from build123d import *

# Parameters (mm, degrees)
SKETCH2_W           = 91.08348254
SKETCH2_H           = 10.16
SKETCH2_R           = 1.75
BOSS_EXTRUDE1_DEPTH = 22.5
CUT_EXTRUDE1_DEPTH  = 88.707853004
FILLET1_R           = 5.08


with BuildPart() as part:
    # Sketch2 → Boss-Extrude1 (new, symmetric)
    with BuildSketch(Plane.XY):
        with Locations((38.619959512, 0)):
            Rectangle(SKETCH2_W, SKETCH2_H)
        with Locations(Location((38.410945338, 0, 0), (0, 0, 180))):
            Circle(SKETCH2_R, mode=Mode.SUBTRACT)
        with Locations(Location((0, 0, 0), (0, 0, 180))):
            Circle(SKETCH2_R, mode=Mode.SUBTRACT)
        with Locations(Location((78.79999988, 0, 0), (0, 0, 180))):
            Circle(SKETCH2_R, mode=Mode.SUBTRACT)
    extrude(amount=BOSS_EXTRUDE1_DEPTH, both=True)

    # Sketch3 → Cut-Extrude1 (cut, through all)
    with BuildSketch(Plane(origin=(0, 5.08, 0), x_dir=(1, 0, 0), z_dir=(0, 1, 0))):
        with BuildLine():
            Line((91.724321271, 17), (72.05824076, 17))
            ThreePointArc((72.05824076, 17), (55.05824076, 0), (72.05824076, -17))
            Line((72.05824076, -17), (91.724321271, -17))
            Line((91.724321271, -17), (91.724321271, 17))
        make_face()
        Polygon((-6.921781758, 15.097756516), (29.791957943, 18.888274186), (45.800007469, 18.888274186), (63.048045595, 22.5), (63.048045595, 41.563803389), (-6.921781758, 41.563803389), align=None)
        with BuildLine():
            Line((-35.26716372, 9.799999958), (7.296822355, 9.799999958))
            ThreePointArc((7.296822355, 9.799999958), (17.096822313, 0), (7.296822355, -9.799999958))
            Line((7.296822355, -9.799999958), (-35.26716372, -9.799999958))
            Line((-35.26716372, -9.799999958), (-35.26716372, 9.799999958))
        make_face()
        Polygon((63.048045595, -22.5), (63.048045595, -41.563803389), (-6.921781758, -41.563803389), (-6.921781758, -15.097756516), (29.791957943, -18.888274186), (45.800007469, -18.888274186), align=None)
    extrude(amount=-CUT_EXTRUDE1_DEPTH, mode=Mode.SUBTRACT)

    # Fillet1
    fillet1_edges = [part.edges().sort_by_distance(p)[0] for p in [
        (-6.921781758, 5.08, -12.448878237),
        (-6.921781758, -5.08, -12.448878237),
        (-6.921781758, -5.08, 12.448878237),
        (-6.921781758, 5.08, 12.448878237),
        (84.161700782, -5.08, -19.75),
        (84.161700782, -5.08, 19.75),
        (84.161700782, 5.08, 19.75),
        (84.161700782, 5.08, -19.75),
    ]]
    fillet(fillet1_edges, radius=FILLET1_R - 0.0001)  # a hair under: the kernel refuses the full size


solid = part.part
Check sheet for the modelled part. Datum: model origin and axes. Units: mm. A direction names the side the tool comes from. Round coordinates to 2 decimals unless told otherwise and drop trailing zeros. Order: outer loops, then holes, each group sorted by start corner. A loop starts at its lowest first (then second) coordinate and runs counter-clockwise, first axis right, second up.
Q1. Set-up check for faces 4 (the face through (2, 0, 9.8)), 5 (the face through (38, 5.08, 0)): record each of +Z, -Z, +X, -X, +Y, -Y from which the full face is reachable in a straight line by a thin tool's end or side.
Filled sheet:
face 4: -X, +Y, -Y
face 5: +Z, -Z, +X, -X, +Y
Q2. Cross-section at D-D, the plane z = 0. Enter the section's corners in (x, y).
Filled sheet:
outline: (17.1, -5.08) - (55.06, -5.08) - (55.06, 5.08) - (17.1, 5.08) - close; hole circle Ø3.5 at (38.41, 0)
Q3. Cross-section at C-C, the plane x = 0. Enter the section's corners in (y, z).
Filled sheet:
outline: (-5.08, -15.81) - (-1.75, -15.81) - (-1.75, -9.8) - (-5.08, -9.8) - close; (-5.08, 9.8) - (-1.75, 9.8) - (-1.75, 15.81) - (-5.08, 15.81) - close; (1.75, -15.81) - (5.08, -15.81) - (5.08, -9.8) - (1.75, -9.8) - close; (1.75, 9.8) - (5.08, 9.8) - (5.08, 15.81) - (1.75, 15.81) - close
Q4. Depth check by flat-ended pin: P1, Ø1, axis at y = 0, z = -6.5, coming from the -X side; P2, Ø3, axis at x = 3, y = 0, coming from the -Z side; P3, Ø3, axis at x = 78.8, y = 0, coming from the -Z side; P4, Ø2, axis at x = 5.5, y = 0, coming from the +Z side. Enter the tip coordinate at first touch or a pass-through.
Filled sheet:
P1: stops at x = 14.16
P2: stops at z = -16.28
P3: passes through
P4: stops at z = 16.48
Q5. Cross-section at A-A, the plane x = 11.5. Enter the section's corners in (y, z), plus the area to 3 significant figures.
Filled sheet:
outline: (-5.08, -17) - (5.08, -17) - (5.08, -8.85) - (-5.08, -8.85) - close; (-5.08, 8.85) - (5.08, 8.85) - (5.08, 17) - (-5.08, 17) - close
area: 166 mm2
Q6. Scan lines: L1, parallel to Y at x = 0, z = -12; L2, parallel to Z at x = 73.5, y = -1.5; L3, parallel to Z at x = 33.5, y = -4.5. Record each from-to range of solid material in increasing order.
Filled sheet:
L1: y = -5.08 to -1.75, 1.75 to 5.08
L2: z = -22.5 to -17, 17 to 22.5
L3: z = -18.89 to 18.89
Q7. Draft check along Z on faces 1 (the face through (80.55, -0.08, 19.71)), 2 (the face through (55.062, 0.071, -0.374)), 3 (the face through (11.178, 0.071, 16.966)). Enter one of: pulls with the +Z half, pulls with the -Z half, needs draft (parallel to the pull), parting line crosses it, or undercut.
Filled sheet:
face 1: needs draft
face 2: undercut
face 3: pulls with the +Z half
Q8. Cross-section at B-B, the plane z = -13.5. Give the number of separate pieces and of enclosed holes in the cut face, plus the area to 3 significant figures.
Filled sheet:
separate pieces: 1
enclosed holes: 2
area: 667 mm2
